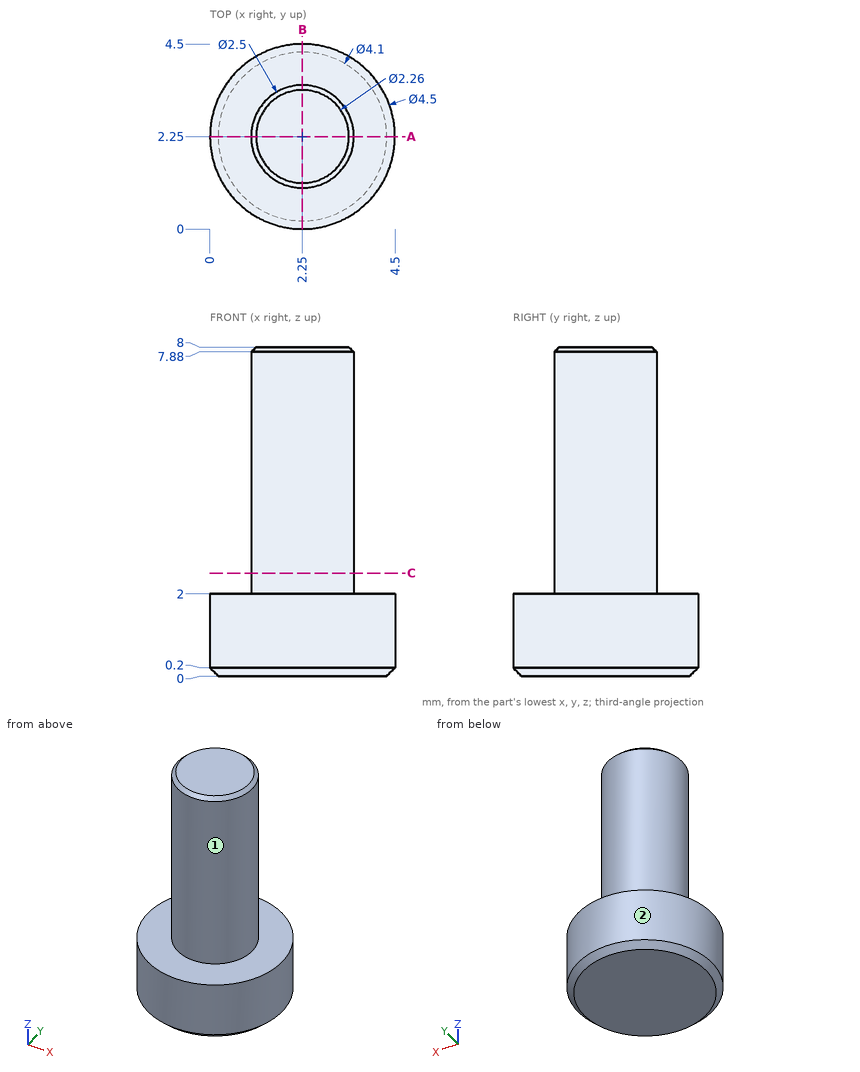
For this review, use the dimensioned drawing (mm, ordinates from the lowest corner) and the shaded views. A direction names the side the tool comes from. Round coordinates to 2 decimals unless told otherwise and drop trailing zeros. Write each loop counter-clockwise with the first axis right and the second up, starting at its lowest first coordinate (ties: lowest second). Pieces come first, ordered by that corner, then holes. Notation, with made-up numbers: M 35,-11 L 82,-11 A21 ccw 82,-2 Z; hole C 5.25,-32.5 d9. An arc over 180 degrees is marked long. Write item = value, one per line. Start each with the question number.
(1) We need section A-A (y = 2.25). Give the boundary of the cut face in (x, z), then the cut area to 3 significant figures.
(2) For line 1 along Z through (x, y) = (2.9, 3.6); line 2 along X through (y, z) = (2.2, 2.75); line 3 along X through (y, z) = (1.15, 5.5), list the stretches that pass through material, from the lowest coordinate up.
(3) Clearance check with flat-ended pins moving along their axes: pin 1 Ø1 at (y, z) = (2, 4) entering from -X; pin 2 Ø2 at (x, z) = (0.5, 1.5) entering from +Y; pin 3 Ø1.5 at (x, z) = (2, 5.5) entering from -Y. State where each tip first meets the part, or that it passes through.
(4) We need section C-C (z = 2.5). Give the boundary of the cut face in (x, y).
(5) For the marked faces 1 and 2, list the 3-axis set-ups (+Z, -Z, +X, -X, +Y, -Y) from which the entire face can be reached by the end or side of a thin tool; tool diameter is ignored.
Results found:
q1.outline = M 0,0.2 L 0.2,0 L 4.3,0 L 4.5,0.2 L 4.5,2 L 3.5,2 L 3.5,7.88 L 3.38,8 L 1.12,8 L 1,7.88 L 1,2 L 0,2 Z
q1.area = 23.9 mm²
q2.line_1 = 0 to 2
q2.line_2 = 1 to 3.5
q2.line_3 = 1.66 to 2.84
q3.pin_1 = 1
q3.pin_2 = 4.37
q3.pin_3 = 1
q4.outline = C 2.25,2.25 d2.5
q5.face_1 = +Z
q5.face_2 = +Z, -Z
